Build history of the part. All positions in model axes, mm. Face numbers are marked on the shaded views. Give positions to 0.01 mm unless a question says otherwise; leave off trailing zeros. Write each loop counter-clockwise with the first axis right and the second up, starting at its lowest first coordinate (ties: lowest second). Pieces come first, ordered by that corner, then holes. Notation, with made-up numbers: (46.25, -24) -> (105.25, -24) arc R25 cw to (105.25, 1) -> close; hole circle Ø7 at (67.25, 18). An arc over 180 degrees is marked (long way). One line per question, with ' | ' between items. Start each with the question number.
(1) Band-saw the part on A-A, the plane z = 3.75. Give the cut face in (x, y) (1 decimal).
(2) Drill centre lines: probe 1 along X at (y, z) = (1, 3.5) (3 decimals); probe 2 along Y at (x, z) = (3.5, -7.5) (3 decimals); probe 3 along Y at (x, z) = (2, -3.75) (3 decimals). Where is each one in solid material? Low to high. Write a range as from..to.
(3) Pull direction Z, two halves, no side cores. Call the marked faces 1, 2 and 3: released by +Z, released by -Z, zero draft, split by the parting line, or undercut.
from build123d import *

# Parameters (mm, degrees)
F0_W     = 19.05
F0_H     = 19.05
F0_R     = 3.96875
F1_DEPTH = 9.525
F6_DEPTH = 19.051


with BuildPart() as f1:
    # F0 (on Top) → F1 (new body)
    with BuildSketch(Plane.XY):
        Rectangle(F0_W, F0_H)
        Circle(F0_R, mode=Mode.SUBTRACT)
    extrude(amount=F1_DEPTH)

    # F4: sweep along a path in F2
    with BuildLine(Plane.XY.offset(9.525)) as f4_path:
        CenterArc((0, 0), 9.525, 0, 360)
    # F3 (on Right) → F4 (sweep, cut)
    with BuildSketch(Plane.YZ):
        Polygon((-14.469163, 8.200215), (-9.525, 9.525), (-14.469163, 9.525), align=None)
    sweep(path=f4_path.line, mode=Mode.SUBTRACT)

    # F5 (on face) → F6 (cut, through all)
    with BuildSketch(Plane.YZ.offset(9.525)):
        Polygon((7.9375, 0), (9.525, 0), (9.525, 1.5875), align=None)
    extrude(amount=-F6_DEPTH, mode=Mode.SUBTRACT)

    # F7: F1 across face


with BuildPart() as f1_1:
    add(f1.part)
    add(f1.part.mirror(Plane(origin=(0, -0.932452, 0), x_dir=(1, 0, 0), z_dir=(0, 0, -1))))


solid = f1_1.part
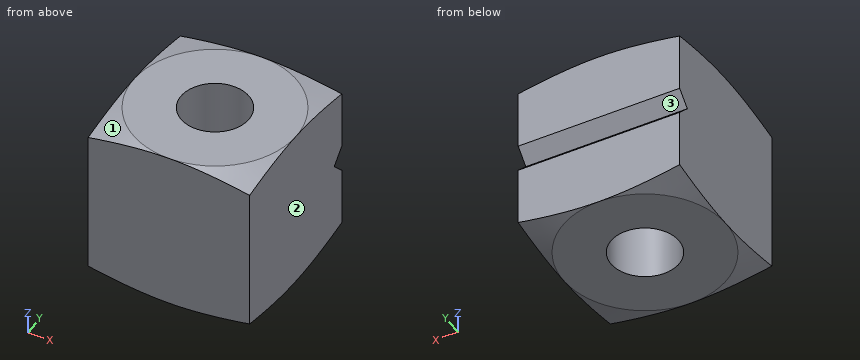
Results:
1) outline: (-9.5, -9.5) -> (9.5, -9.5) -> (9.5, 9.5) -> (-9.5, 9.5) -> close; hole circle Ø7.9 at (0, 0)
2) probe 1: x = -9.525..-3.841, 3.841..9.525 | probe 2: y = -9.525..-1.871, 1.871..9.525 | probe 3: y = -9.525..-3.428, 3.428..9.525
3) face 1: released by +Z | face 2: zero draft | face 3: undercut
